Geometry check sheet. Reference: the model listing, model coordinates, mm. Give positions to 0.01 mm unless a question says otherwise; leave off trailing zeros. Loops run counter-clockwise (first coordinate to the right, second up) from the corner with the lowest first, then second, coordinate; pieces in that order, holes last. Notation, with made-up numbers: (80.25, 27) -> (113.25, 27) arc R27 cw to (113.25, 47) -> close; hole circle Ø5 at (-2, 14.5). An arc over 180 degrees is marked (long way). Answer in a Markdown table with one row per item. Add a question column.
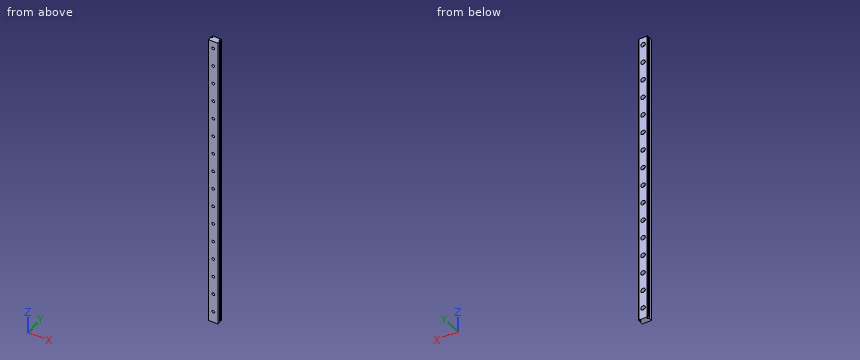
```python
from build123d import *

# Parameters (mm, degrees)
BOSS_EXTRUDE2_DEPTH = 400
FILLET5_R           = 0.5
SKETCH3_R           = 3
CUT_EXTRUDE2_DEPTH  = 4.5
SKETCH4_R           = 1.75
CUT_EXTRUDE3_DEPTH  = 14.5
SKETCH5_W           = 12
SKETCH5_H           = 4.057387372
CUT_EXTRUDE4_DEPTH  = 682.5


with BuildPart() as part:
    # Sketch1 → Boss-Extrude2 (new body)
    with BuildSketch(Plane.XY):
        Polygon((0, 0), (12, 0), (12, 8.403449878), (9.5, 9.846825551), (12, 11.290201224), (12, 12), (0, 12), (0, 11.290201224), (2.5, 9.846825551), (0, 8.403449878), align=None)
    extrude(amount=BOSS_EXTRUDE2_DEPTH)

    # Fillet5
    # the kernel refuses this fillet: 0.5 mm, written as the material it adds along each edge
    with BuildSketch(Plane(origin=(2.5, 9.846825551, 0), x_dir=(-0.8660254037844382, 0.5000000000000009, 0), z_dir=(0, 0, 1)), Plane(origin=(9.5, 9.846825551, 0), x_dir=(0.8660254037844379, -0.5000000000000013, 0), z_dir=(0, 0, 1))) as fillet5_piece_1:
        with BuildLine():
            CenterArc((FILLET5_R * 1.73205080757, FILLET5_R), FILLET5_R, 150, 120)
            Line((FILLET5_R * 0.866025403784, FILLET5_R * 1.5), (0, 0))
            Line((0, 0), (FILLET5_R * 1.73205080757, 0))
        make_face()
    extrude(amount=400)
    # the kernel refuses this fillet: 0.5 mm, written as the material it takes off along each edge
    with BuildSketch(Plane(origin=(0, 8.403449878, -0.721687836), x_dir=(0, -1, 0), z_dir=(0, 0, 1))) as fillet5_2_piece_1:
        with BuildLine():
            CenterArc((FILLET5_R * 0.57735026919, FILLET5_R), FILLET5_R, 210, 60)
            Line((-FILLET5_R * 0.288675134595, FILLET5_R * 0.5), (0, 0))
            Line((0, 0), (FILLET5_R * 0.57735026919, 0))
        make_face()
    extrude(amount=401.443375673, mode=Mode.SUBTRACT)
    with BuildSketch(Plane(origin=(0, 11.290201224, -0.721687836), x_dir=(0, 1, 0), z_dir=(0, 0, 1)), Plane(origin=(12, 11.290201224, -0.721687836), x_dir=(-0.8660254037844355, -0.5000000000000052, 0), z_dir=(0, 0, 1)), Plane(origin=(12, 8.403449878, -0.721687836), x_dir=(0, -1, 0), z_dir=(0, 0, 1))) as fillet5_2_piece_2:
        with BuildLine():
            CenterArc((FILLET5_R * 0.57735026919, -FILLET5_R), FILLET5_R, 90, 60)
            Line((-FILLET5_R * 0.288675134595, -FILLET5_R * 0.5), (0, 0))
            Line((0, 0), (FILLET5_R * 0.57735026919, 0))
        make_face()
    extrude(amount=401.443375673, mode=Mode.SUBTRACT)
    with BuildSketch(Plane(origin=(0, 12, -1.25), x_dir=(1, 0, 0), z_dir=(0, 0, 1)), Plane(origin=(12, 12, -1.25), x_dir=(0, -1, 0), z_dir=(0, 0, 1))) as fillet5_2_piece_3:
        with BuildLine():
            CenterArc((FILLET5_R, -FILLET5_R), FILLET5_R, 90, 90)
            Line((0, -FILLET5_R), (0, 0))
            Line((0, 0), (FILLET5_R, 0))
        make_face()
    extrude(amount=402.5, mode=Mode.SUBTRACT)

    # Sketch3 → Cut-Extrude2 (cut)
    with BuildSketch(Plane(origin=(0, 12, 0), x_dir=(1, 0, 0), z_dir=(0, 1, 0))):
        with Locations((6, -490)):
            Circle(SKETCH3_R)
        with Locations((6, -440)):
            Circle(SKETCH3_R)
        with Locations((6, -415)):
            Circle(SKETCH3_R)
        with Locations(Location((6, -390, 0), (0, 0, 180))):
            Circle(SKETCH3_R)
        with Locations(Location((6, -365, 0), (0, 0, 180))):
            Circle(SKETCH3_R)
        with Locations(Location((6, -340, 0), (0, 0, 180))):
            Circle(SKETCH3_R)
        with Locations(Location((6, -315, 0), (0, 0, 180))):
            Circle(SKETCH3_R)
        with Locations(Location((6, -290, 0), (0, 0, 180))):
            Circle(SKETCH3_R)
        with Locations(Location((6, -265, 0), (0, 0, 180))):
            Circle(SKETCH3_R)
        with Locations(Location((6, -240, 0), (0, 0, 180))):
            Circle(SKETCH3_R)
        with Locations(Location((6, -215, 0), (0, 0, 180))):
            Circle(SKETCH3_R)
        with Locations(Location((6, -190, 0), (0, 0, 180))):
            Circle(SKETCH3_R)
        with Locations(Location((6, -165, 0), (0, 0, 180))):
            Circle(SKETCH3_R)
        with Locations(Location((6, -140, 0), (0, 0, 180))):
            Circle(SKETCH3_R)
        with Locations(Location((6, -115, 0), (0, 0, 180))):
            Circle(SKETCH3_R)
        with Locations(Location((6, -90, 0), (0, 0, 180))):
            Circle(SKETCH3_R)
        with Locations(Location((6, -65, 0), (0, 0, 180))):
            Circle(SKETCH3_R)
        with Locations(Location((6, -40, 0), (0, 0, 180))):
            Circle(SKETCH3_R)
        with Locations(Location((6, -15, 0), (0, 0, 180))):
            Circle(SKETCH3_R)
        with Locations((6, -465)):
            Circle(SKETCH3_R)
    extrude(amount=-CUT_EXTRUDE2_DEPTH, mode=Mode.SUBTRACT)

    # Sketch4 → Cut-Extrude3 (cut)
    with BuildSketch(Plane(origin=(0, 12, 0), x_dir=(1, 0, 0), z_dir=(0, 1, 0))):
        with Locations(Location((6, -15, 0), (0, 0, 180))):
            Circle(SKETCH4_R)
        with Locations(Location((6, -40, 0), (0, 0, 180))):
            Circle(SKETCH4_R)
        with Locations(Location((6, -65, 0), (0, 0, 180))):
            Circle(SKETCH4_R)
        with Locations(Location((6, -90, 0), (0, 0, 180))):
            Circle(SKETCH4_R)
        with Locations(Location((6, -115, 0), (0, 0, 180))):
            Circle(SKETCH4_R)
        with Locations(Location((6, -140, 0), (0, 0, 180))):
            Circle(SKETCH4_R)
        with Locations(Location((6, -165, 0), (0, 0, 180))):
            Circle(SKETCH4_R)
        with Locations(Location((6, -190, 0), (0, 0, 180))):
            Circle(SKETCH4_R)
        with Locations(Location((6, -215, 0), (0, 0, 180))):
            Circle(SKETCH4_R)
        with Locations(Location((6, -240, 0), (0, 0, 180))):
            Circle(SKETCH4_R)
        with Locations(Location((6, -265, 0), (0, 0, 180))):
            Circle(SKETCH4_R)
        with Locations(Location((6, -290, 0), (0, 0, 180))):
            Circle(SKETCH4_R)
        with Locations(Location((6, -315, 0), (0, 0, 180))):
            Circle(SKETCH4_R)
        with Locations(Location((6, -340, 0), (0, 0, 180))):
            Circle(SKETCH4_R)
        with Locations(Location((6, -365, 0), (0, 0, 180))):
            Circle(SKETCH4_R)
        with Locations(Location((6, -390, 0), (0, 0, 180))):
            Circle(SKETCH4_R)
        with Locations((6, -415)):
            Circle(SKETCH4_R)
        with Locations((6, -440)):
            Circle(SKETCH4_R)
        with Locations((6, -465)):
            Circle(SKETCH4_R)
        with Locations((6, -490)):
            Circle(SKETCH4_R)
    extrude(amount=-CUT_EXTRUDE3_DEPTH, mode=Mode.SUBTRACT)

    # Sketch5 → Cut-Extrude4 (cut)
    with BuildSketch(Plane(origin=(0, 0, 0), x_dir=(-1, 0, 0), z_dir=(0, 0, -1))):
        with Locations((-6, 2.028693686)):
            Rectangle(SKETCH5_W, SKETCH5_H)
    extrude(amount=-CUT_EXTRUDE4_DEPTH, mode=Mode.SUBTRACT)


solid = part.part
```
1. Sectioned sample at A-A (z = 233). Enter the section's corners in (x, y), plus the area to 3 significant figures.
2. Material ranges on L1, parallel to X at y = 11.75, z = 133; L2, parallel to X at y = 6.35, z = 190; L3, parallel to X at y = 11.5, z = 261, recorded low to high. Write a range as from..to.
3. Gauge pin test, flat end, axial feed: pin 1 Ø5 at (x, z) = (6, 190) entering from +Y. Record the tip position at first contact, or that the pin passes through.
Response:
| question | item | result |
|---|---|---|
| 1 | outline | (0, 4.06) -> (12, 4.06) -> (12, 8.11) arc R0.5 ccw to (11.75, 8.55) -> (10.25, 9.41) arc R0.5 cw to (10.25, 10.28) -> (11.75, 11.15) arc R0.5 ccw to (12, 11.54) arc R0.5 ccw to (11.5, 12) -> (0.5, 12) arc R0.5 ccw to (0, 11.54) arc R0.5 ccw to (0.25, 11.15) -> (1.75, 10.28) arc R0.5 cw to (1.75, 9.41) -> (0.25, 8.55) arc R0.5 ccw to (0, 8.11) -> close |
| 1 | area | 88.3 mm2 |
| 2 | L1 | x = 0.07..11.93 |
| 2 | L2 | x = 0..4.25, 7.75..12 |
| 2 | L3 | x = 0.01..11.99 |
| 3 | pin 1 | stops at y = 7.5 |
